Design review of the part built by this model. Coordinates are the model's own, in mm. Round coordinates to 2 decimals unless told otherwise and drop trailing zeros. Write each loop counter-clockwise with the first axis right and the second up, starting at its lowest first coordinate (ties: lowest second). Pieces come first, ordered by that corner, then holes. Notation, with made-up numbers: M 76,8 L 117,8 A14 ccw 117,22 Z; hole C 63.25,-11 d9. An arc over 180 degrees is marked long. One line per question, with ' | ' between items. Start each with the question number.
Item 1: Insertion check: pin 1 Ø1 at (y, z) = (2, -0.5) entering from +X; pin 2 Ø3 at (y, z) = (1, 2.5) entering from +X. Each pin has a flat end and moves straight along its axis. Give the tip position at first contact, or say it passes through.
Item 2: For L1, parallel to Z at x = -0.5, y = 2.05; L2, parallel to Z at x = 1, y = 0.6; L3, parallel to Y at x = 0.5, z = -3.5, list the stretches that pass through material, from the lowest coordinate up.
Item 3: Add section C-C, the plane y = 4.35. State the section outline as (x, z) points.
Item 4: Add section D-D, the plane y = 2.3. State the section outline as (x, z) points.
Item 5: Draft analysis for pull direction Z (two halves, no side actions). For faces 1 (the face through (-0.72, 3.4, 2.27)), 2 (the face through (3.905, 4.659, -0.867)), 3 (the face through (2, 5.5, 2)), state which applies: released by +Z, released by -Z, zero draft, split by the parting line, or undercut.
Item 6: Add section A-A, the plane x = 0. State the section outline as (y, z) points, and give its area (3 significant figures).
Item 7: Add section B-B, the plane z = 0. State the section outline as (x, y) points, and give its area (3 significant figures).
```python
from build123d import *
from OCP.BRepFilletAPI import BRepFilletAPI_MakeChamfer

# Parameters (mm, degrees)
CHAMFER1_SIZE  = 0.2
CHAMFER1_SIZE2 = 0.248451997


with BuildPart() as part:
    # Sketch1 → Revolve1 (revolve)
    with BuildSketch(Plane.XY, mode=Mode.PRIVATE) as revolve1_sk:
        Polygon((-3, 0), (-3.5, 0), (-3.5, 4), (-4, 4), (-4, 5.5), (-2, 5.5), align=None)
    revolve(revolve1_sk.sketch.rotate(Axis((0, 5.5, 0), (0, -1, 0)), 270), axis=Axis((0, 5.5, 0), (0, -1, 0)))

    # Chamfer1: one chamfer whose edges measure the first distance from different faces: ONE call of the kernel's chamfer builder (chamfer() names one face for all edges)
    chamfer1_edges_1 = [part.edges().sort_by_distance(p)[0] for p in [
        (0, 5.5, -4),
    ]]
    chamfer1_edges_2 = [part.edges().sort_by_distance(p)[0] for p in [
        (0, 0, -3),
    ]]
    chamfer1_side_2 = [part.faces().sort_by_distance(p)[0] for p in [
        (0, 2.75, -2.5),
    ]]
    chamfer1 = BRepFilletAPI_MakeChamfer(part.part.solid().wrapped)
    for e in chamfer1_edges_1:
        chamfer1.Add(CHAMFER1_SIZE, e.wrapped)
    for e in chamfer1_edges_2:
        chamfer1.Add(CHAMFER1_SIZE, CHAMFER1_SIZE2, e.wrapped, chamfer1_side_2[0].wrapped)  # the first distance lies on this face
    add(Compound.cast(chamfer1.Shape()), mode=Mode.REPLACE)


solid = part.part
```
Computed values:
1) pin 1: stops at x = 3.5 | pin 2: stops at x = 3.35
2) L1: z = -3.46 to -2.58, 2.58 to 3.46 | L2: z = -3.35 to -2.71, 2.71 to 3.35 | L3: y = 4 to 5.5
3) outline: C 0,0 d8; hole C 0,0 d4.42
4) outline: C 0,0 d7; hole C 0,0 d5.16
5) face 1: undercut | face 2: split by the parting line | face 3: zero draft
6) outline: M 0,-3.5 L 4,-3.5 L 4,-4 L 5.3,-4 L 5.5,-3.8 L 5.5,-2 L 0.2,-2.96 L 0,-3.25 Z; M 0,3.25 L 0.2,2.96 L 5.5,2 L 5.5,3.8 L 5.3,4 L 4,4 L 4,3.5 L 0,3.5 Z | area: 12.4 mm^2
7) outline: M -4,4 L -3.5,4 L -3.5,0 L -3.25,0 L -2.96,0.2 L -2,5.5 L -3.8,5.5 L -4,5.3 Z; M 2,5.5 L 2.96,0.2 L 3.25,0 L 3.5,0 L 3.5,4 L 4,4 L 4,5.3 L 3.8,5.5 Z | area: 12.4 mm^2
